Model file for the job. Use its own axes, mm. A direction names the side the tool comes from. Give positions to 0.01 mm unless a question says otherwise; leave off trailing zeros. Write each loop counter-clockwise with the first axis right and the second up, starting at its lowest first coordinate (ties: lowest second). Pieces come first, ordered by that corner, then holes. Notation, with made-up numbers: (58.25, 47) - (75.25, 47) arc R20 cw to (75.25, 54) - close; hole circle Ø6 at (74.25, 29.25). An arc over 180 degrees is marked (long way). One line per item, written item: value. Start each with the question number.
(1) Cut at B-B, the plane z = 0. State how many separate pieces and enclosed holes the cut face has, and give its area (3 significant figures).
(2) 3-axis set-ups, long thin cutter, end or side, ignore diameter. For faces 1 (the face through (0, 3, 7.1)), 2 (the face through (37, 3, 6.955)), 3 (the face through (30, 5.746, 0)), 4 (the face through (37, 3, -6.955)), 5 (the face through (0, 6.125, -12)): which of +Z, -Z, +X, -X, +Y, -Y reach the whole face in a straight line?
(3) Mould opens along X. For faces 6 (the face through (0, 3, -7.1)), 7 (the face through (0, 6.125, 12)), 8 (the face through (38.14, 3, 0)) say: pulls with the +X half, pulls with the -X half, needs draft (parallel to the pull), parting line crosses it, or undercut.
(4) Probe L1, parallel to X at y = 1.8, z = 0 (3 decimals); L2, parallel to Z at x = 2.5, y = 6; L3, parallel to X at y = 3, z = -12.5. List the from-to ranges inside material, lowest first.
(5) Drop a flat-ended pin along its axis: P1, Ø4, axis at x = 33, z = -8.5, coming from the +Y side. Give the stop position or say it passes through.
(6) Cut at A-A, the plane x = -2. List the corners of the cut face in (y, z) (3 decimals).
from build123d import *

# Parameters (mm, degrees)
SKETCH_1_W                = 50.28
SKETCH_1_H                = 34.2
SKETCH_1_W_2              = 30.28
SKETCH_1_H_2              = 14.2
EXTRUDE_1_DEPTH           = 12.25
SKETCH_4_W                = 13
SKETCH_4_H                = 13.91
EXTRUDE_1_2_DEPTH         = 74.82
SKETCH_5_W                = 13.91
SKETCH_5_H                = 16.23
EXTRUDE_2_DEPTH           = 16
SKETCH_7_R                = 25.25
SKETCH_7_R_2              = 15.25
EXTRUDE_2_2_DEPTH         = 16.23
SKETCH_15_R               = 1.91
CUT_EXTRUDE_6_DEPTH       = 97.964478439
SKETCH_16_W               = 13.91
SKETCH_16_H               = 16.23
EXTRUDE_4_DEPTH           = 10
SKETCH_17_R               = 1.91
CUT_EXTRUDE_7_DEPTH       = 102.16913771
SKETCH_18_W               = 49.344544624
SKETCH_18_H               = 6.125
CUT_EXTRUDE_8_DEPTH       = 105.840616652
SKETCH_19_W               = 34.2
SKETCH_19_H               = 6.125
CUT_EXTRUDE_9_DEPTH       = 10
SKETCH_21_R               = 1.91
CUT_EXTRUDE_10_DEPTH      = 10
SKETCH_20_R               = 1.91
CUT_EXTRUDE_11_DEPTH      = 10
FILLET_START              = -7.1
FILLET_1_DEPTH            = 14.2
FILLET_2_DEPTH            = 14.2
SKETCH_29_W               = 13.91
SKETCH_29_H               = 74.82
EXTRUDE_5_DEPTH           = 10
SKETCH_30_W               = 10
SKETCH_30_H               = 58.59
CUT_EXTRUDE_13_DEPTH      = 102.16913771
SKETCH_32_W               = 34.2
SKETCH_32_H               = 5.745736365
EXTRUDE_6_DEPTH           = 10
CUT_EXTRUDE_16_DEPTH      = 50
CUT_EXTRUDE_16_DEPTH_BACK = 50
SKETCH_38_W               = 116.985630298
SKETCH_38_H               = 80.538350638
SKETCH_41_W               = 13.91
SKETCH_41_H               = 5.745736365
EXTRUDE_7_DEPTH           = 3


with BuildPart() as part:
    # 草圖1 → Extrude 1 (new body)
    with BuildSketch(Plane(origin=(0, 0, 0), x_dir=(1, 0, 0), z_dir=(0, 1, 0))):
        Rectangle(SKETCH_1_W, SKETCH_1_H)
        Rectangle(SKETCH_1_W_2, SKETCH_1_H_2, mode=Mode.SUBTRACT)
    extrude(amount=EXTRUDE_1_DEPTH)

    # 草圖4 → Extrude 1 2 (add)
    with BuildSketch(Plane.XZ):
        with Locations((18.64, 0)):
            Rectangle(SKETCH_4_W, SKETCH_4_H)
    extrude(amount=EXTRUDE_1_2_DEPTH)

    # 草圖5 → Extrude 2 (add)
    with BuildSketch(Plane.ZY.offset(-12.14)):
        with Locations((0, -66.705)):
            Rectangle(SKETCH_5_W, SKETCH_5_H)
    extrude(amount=EXTRUDE_2_DEPTH)

    # 草圖7 → Extrude 2 2 (add)
    with BuildSketch(Plane(origin=(3.626674765, -74.82, 0), x_dir=(1, 0, 0), z_dir=(0, -1, 0))):
        with Locations((-30.978154344, 0)):
            Circle(SKETCH_7_R)
        with Locations((-30.978154344, 0)):
            Circle(SKETCH_7_R_2, mode=Mode.SUBTRACT)
    extrude(amount=-EXTRUDE_2_2_DEPTH)

    # 草圖15 → 除料-伸長6 (cut, through all)
    with BuildSketch(Plane(origin=(0, 0, -6.955), x_dir=(-1, 0, 0), z_dir=(0, 0, -1))):
        with Locations((-4.530883248, -66.705)):
            Circle(SKETCH_15_R)
    extrude(amount=-CUT_EXTRUDE_6_DEPTH, mode=Mode.SUBTRACT)

    # 草圖16 → 填料-伸長4 (add)
    with BuildSketch(Plane(origin=(-60, 0, 0), x_dir=(0, 0, -1), z_dir=(1, 0, 0))):
        with Locations((0, -66.705)):
            Rectangle(SKETCH_16_W, SKETCH_16_H)
    extrude(amount=EXTRUDE_4_DEPTH)

    # 草圖17 → 除料-伸長7 (cut, through all)
    with BuildSketch(Plane(origin=(0, 0, -6.955), x_dir=(-1, 0, 0), z_dir=(0, 0, -1))):
        with Locations((55.812362827, -66.705)):
            Circle(SKETCH_17_R)
    extrude(amount=-CUT_EXTRUDE_7_DEPTH, mode=Mode.SUBTRACT)

    # 草圖18 → 除料-伸長8 (cut, through all)
    with BuildSketch(Plane(origin=(0, 0, -17.1), x_dir=(-1, 0, 0), z_dir=(0, 0, -1))):
        with Locations((0.467727688, 9.1875)):
            Rectangle(SKETCH_18_W, SKETCH_18_H)
    extrude(amount=-CUT_EXTRUDE_8_DEPTH, mode=Mode.SUBTRACT)

    # 草圖19 → 除料-伸長9 (cut)
    with BuildSketch(Plane.ZY.offset(-24.204544624)):
        with Locations((0, 9.1875)):
            Rectangle(SKETCH_19_W, SKETCH_19_H)
    extrude(amount=-CUT_EXTRUDE_9_DEPTH, mode=Mode.SUBTRACT)

    # 草圖21 → 除料-伸長10 (cut)
    with BuildSketch(Plane(origin=(0, 6.125, 0), x_dir=(1, 0, 0), z_dir=(0, 1, 0))):
        with Locations(Location((17.69, 0, 0), (0, 0, 270))):
            Circle(SKETCH_21_R)
    extrude(amount=-CUT_EXTRUDE_10_DEPTH, mode=Mode.SUBTRACT)

    # 草圖20 → 除料-伸長11 (cut)
    with BuildSketch(Plane(origin=(0, 6.125, 0), x_dir=(1, 0, 0), z_dir=(0, 1, 0))):
        with Locations(Location((-17.395, 0, 0), (0, 0, 270))):
            Circle(SKETCH_20_R)
    extrude(amount=-CUT_EXTRUDE_11_DEPTH, mode=Mode.SUBTRACT)

    # 圓角1: read off the stored shape, not the designer's step
    # 圓角1 outline → 圓角1 (cut)
    with BuildSketch(Plane.XY.offset(FILLET_START)):
        with BuildLine():
            add(Edge.make_bspline(
                [(-15.14, 0), (-21.974170252, 5.199829476), (-25.14, 5.745736365)],
                knots=[0, 0, 0, 0.664102345, 0.664102345, 0.664102345], degree=2, weights=[1, 2.223777218, 1.822127795]))
            Line((-15.14, 0), (-15.14, 6.125))
            Line((-15.14, 6.125), (-25.14, 6.125))
            Line((-25.14, 6.125), (-25.14, 5.745736365))
        make_face()
    extrude(amount=FILLET_1_DEPTH, mode=Mode.SUBTRACT)

    # 圓角2: read off the stored shape, not the designer's step
    # 圓角2 outline → 圓角2 (cut)
    with BuildSketch(Plane.XY.offset(FILLET_START)):
        with BuildLine():
            Line((15.14, 6.125), (15.14, 0))
            add(Edge.make_bspline(
                [(15.14, 0), (21.974170252, 5.199829476), (25.14, 5.745736365)],
                knots=[0, 0, 0, 0.664102345, 0.664102345, 0.664102345], degree=2, weights=[1, 2.223777218, 1.822127795]))
            Line((25.14, 5.745736365), (25.14, 6.125))
            Line((25.14, 6.125), (15.14, 6.125))
        make_face()
    extrude(amount=FILLET_2_DEPTH, mode=Mode.SUBTRACT)

    # 草圖29 → 填料-伸長5 (add)
    with BuildSketch(Plane(origin=(25.14, 0, 0), x_dir=(0, 0, -1), z_dir=(1, 0, 0))):
        with Locations((0, -37.41)):
            Rectangle(SKETCH_29_W, SKETCH_29_H)
    extrude(amount=EXTRUDE_5_DEPTH)

    # 草圖30 → 除料-伸長13 (cut, through all)
    with BuildSketch(Plane.XY.offset(6.955)):
        with Locations((17.14, -29.295)):
            Rectangle(SKETCH_30_W, SKETCH_30_H)
    extrude(amount=-CUT_EXTRUDE_13_DEPTH, mode=Mode.SUBTRACT)

    # 草圖32 → 填料-伸長6 (add)
    with BuildSketch(Plane(origin=(25.14, 0, 0), x_dir=(0, 0, -1), z_dir=(1, 0, 0))):
        with Locations((0, 2.872868182)):
            Rectangle(SKETCH_32_W, SKETCH_32_H)
    extrude(amount=EXTRUDE_6_DEPTH)

    # 草圖38 → 除料-伸長16 (cut, two sides: drawn at the far end of the back side and taken through both)
    with BuildSketch(Plane(origin=(0, 0, -6.955), x_dir=(-1, 0, 0), z_dir=(0, 0, -1)).offset(-CUT_EXTRUDE_16_DEPTH_BACK)):
        with Locations((7.268869252, -40.269175319)):
            Rectangle(SKETCH_38_W, SKETCH_38_H)
    extrude(amount=CUT_EXTRUDE_16_DEPTH + CUT_EXTRUDE_16_DEPTH_BACK, mode=Mode.SUBTRACT)

    # 草圖41 → 填料-伸長7 (add)
    with BuildSketch(Plane(origin=(35.14, 0, 0), x_dir=(0, 0, -1), z_dir=(1, 0, 0))):
        with Locations((0, 2.872868182)):
            Rectangle(SKETCH_41_W, SKETCH_41_H)
    extrude(amount=EXTRUDE_7_DEPTH)


solid = part.part
Answers follow:
1. separate pieces: 4
1. enclosed holes: 0
1. area: 129 mm²
2. face 1: +Y
2. face 2: +Z, +X, +Y, -Y
2. face 3: +Z, -Z, +X, +Y
2. face 4: -Z, +X, +Y, -Y
2. face 5: +Z, -Z, +X, -X, +Y
3. face 6: undercut
3. face 7: needs draft
3. face 8: pulls with the +X half
4. L1: x = -25.14 to -19.305, 19.6 to 38.14
4. L2: z = -17.1 to -7.1, 7.1 to 17.1
4. L3: x = -25.14 to 35.14
5. P1: stops at y = 5.75
6. outline: (0, -17.1) - (6.125, -17.1) - (6.125, -7.1) - (0, -7.1) - close; (0, 7.1) - (6.125, 7.1) - (6.125, 17.1) - (0, 17.1) - close
